The model under review builds one solid part; all positions refer to its coordinate system, in mm. Face numbers are marked on the shaded views. A direction names the side the tool comes from. Give positions to 0.01 mm unless a question says otherwise; leave off trailing zeros. Loops run counter-clockwise (first coordinate to the right, second up) from the corner with the lowest first, then second, coordinate; pieces in that order, holes last. Notation, with made-up numbers: M 20,-20 L 35,-20 A24 ccw 35,-7 Z; hole C 40.25,-23.5 d10. An arc over 180 degrees is marked long. One line per item, written item: value. Start each with the question number.
Q1. For the marked faces 1, 2 and 3, list the 3-axis set-ups (+Z, -Z, +X, -X, +Y, -Y) from which the entire face can be reached by the end or side of a thin tool; tool diameter is ignored.
Q2. We need section A-A on x = -83. Write out the cut boundary in (y, z).
Q3. We need section B-B on y = 8. Write out the cut boundary in (x, z).
Q4. Mouldability with a two-part tool opening along Y and no side actions: class the marked faces 4, 5 and 6 as released by +Y, released by -Y, zero draft, split by the parting line, or undercut.
Q5. For pin 1 (8 mm diameter, centred on x = -107, z = -29, fed in from +Y); pin 2 (15.5 mm diameter, centred on y = -14, z = 3.5, fed in from +X); pin 3 (5.5 mm diameter, centred on y = -68.5, z = 13.5, fed in from +X), all flat-tipped, find the tip position at first contact; note any pin that passes through.
Q6. We need section D-D on x = -66.5. Write out the cut boundary in (y, z), plus the area to 3 significant figures.
Q7. We need section C-C on z = -4. Write out the cut boundary in (x, y).
Q8. To check wall thickness, follow line 1 along Z through (x, y) = (-26.5, 23.5); line 2 along X through (y, z) = (1, 17); line 3 along X through (y, z) = (-15.5, 6). State the ranges of each line that lie inside material, in increasing order. Write a range as from..to.
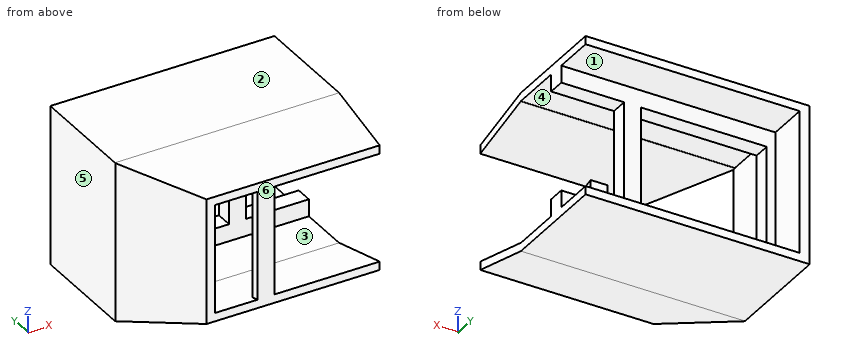
```python
from build123d import *

# Parameters (mm, degrees)
SKETCH1_W                = 74
SKETCH1_H                = 64
BOSS_EXTRUDE3_DEPTH      = 10
BOSS_EXTRUDE4_DEPTH      = 24
BOSS_EXTRUDE4_DEPTH_BACK = 80
SKETCH3_W                = 264
SKETCH3_H                = 94
SKETCH3_W_2              = 252.2
SKETCH3_H_2              = 84.2
SKETCH4_W                = 264
SKETCH4_H                = 94
SKETCH4_W_2              = 194
SKETCH4_H_2              = 64
BOSS_EXTRUDE5_DEPTH      = 40
CHAMFER4_SIZE            = 39.811344649
CHAMFER4_SIZE_2          = 30
CHAMFER7_SIZE            = 39.811344649
CHAMFER7_SIZE_2          = 30
CHAMFER8_SIZE            = 10
CHAMFER8_SIZE_2          = 40.107809335
CHAMFER9_SIZE            = 40.107809335
CHAMFER9_SIZE_2          = 10
SKETCH7_W                = 10
SKETCH7_H                = 74
BOSS_EXTRUDE6_DEPTH      = 5


with BuildPart() as part:
    # Sketch1 → Boss-Extrude3 (new body)
    with BuildSketch(Plane(origin=(0, 0, 0), x_dir=(1, 0, 0), z_dir=(0, 1, 0))):
        Polygon((-47, 42.1), (-126.1, 42.1), (-126.1, -42.1), (-47, -42.1), (-37, -42.1), (37, -42.1), (47, -42.1), (126.1, -42.1), (126.1, 42.1), (47, 42.1), (37, 42.1), (-37, 42.1), align=None)
        with Locations((-84, 0)):
            Rectangle(SKETCH1_W, SKETCH1_H, mode=Mode.SUBTRACT)
        Rectangle(SKETCH1_W, SKETCH1_H, mode=Mode.SUBTRACT)
        with Locations((84, 0)):
            Rectangle(SKETCH1_W, SKETCH1_H, mode=Mode.SUBTRACT)
    extrude(amount=BOSS_EXTRUDE3_DEPTH)

    # Sketch3 → Boss-Extrude4 (add, two sides: drawn at the far end of the back side and taken through both)
    with BuildSketch(Plane(origin=(0, 10, 0), x_dir=(1, 0, 0), z_dir=(0, 1, 0)).offset(-BOSS_EXTRUDE4_DEPTH_BACK)):
        Rectangle(SKETCH3_W, SKETCH3_H)
        Rectangle(SKETCH3_W_2, SKETCH3_H_2, mode=Mode.SUBTRACT)
    extrude(amount=BOSS_EXTRUDE4_DEPTH + BOSS_EXTRUDE4_DEPTH_BACK)

    # Sketch4 → Boss-Extrude5 (add)
    with BuildSketch(Plane(origin=(0, -70, 0), x_dir=(-1, 0, 0), z_dir=(0, -1, 0))):
        Rectangle(SKETCH4_W, SKETCH4_H)
        Rectangle(SKETCH4_W_2, SKETCH4_H_2, mode=Mode.SUBTRACT)
    extrude(amount=-BOSS_EXTRUDE5_DEPTH)

    # Chamfer4
    # the kernel refuses this chamfer: 39.811344649, 30 mm, written as the material it takes off along each edge
    with BuildSketch(Plane(origin=(-132, -70, 149.735778307), x_dir=(-0.023321052992758384, 0.9997280272590686, 0), z_dir=(0, 0, -1))) as chamfer4_piece_1:
        Polygon((CHAMFER4_SIZE * 0.999728027249, CHAMFER4_SIZE * 0.0233210529925), (-CHAMFER4_SIZE_2 * 0.0233210529928, CHAMFER4_SIZE_2 * 0.999728027259), (0, 0), align=None)
    extrude(amount=299.471556613, mode=Mode.SUBTRACT)
    with BuildSketch(Plane(origin=(-97, -30, 32), x_dir=(-0.9991572559820394, 0.04104604510109794, 0), z_dir=(0, 0, -1))) as chamfer4_piece_2_section:
        Polygon((CHAMFER4_SIZE_2 * 0.999157255982, -CHAMFER4_SIZE_2 * 0.0410460451011), (-CHAMFER4_SIZE * 0.0410460451007, -CHAMFER4_SIZE * 0.999157255972), (0, 0), align=None)
    chamfer4_piece_2 = extrude(amount=64, mode=Mode.PRIVATE)
    chamfer4_piece_2 = split(chamfer4_piece_2, bisect_by=Plane(origin=(-126.1, -43.282043753, 0), z_dir=(1, 0, 0)), keep=Keep.TOP, mode=Mode.PRIVATE)
    add(chamfer4_piece_2, mode=Mode.SUBTRACT)

    # Chamfer7
    # the kernel refuses this chamfer: 39.811344649, 30 mm, written as the material it takes off along each edge
    with BuildSketch(Plane(origin=(132, -70, -149.735778307), x_dir=(0.02332105299275837, 0.9997280272590686, 0), z_dir=(0, 0, 1))) as chamfer7_piece_1:
        Polygon((CHAMFER7_SIZE * 0.999728027249, CHAMFER7_SIZE * 0.0233210529925), (-CHAMFER7_SIZE_2 * 0.0233210529928, CHAMFER7_SIZE_2 * 0.999728027259), (0, 0), align=None)
    extrude(amount=299.471556613, mode=Mode.SUBTRACT)
    with BuildSketch(Plane(origin=(97, -30, -32), x_dir=(0.9991572559820394, 0.04104604510109794, 0), z_dir=(0, 0, 1))) as chamfer7_piece_2_section:
        Polygon((CHAMFER7_SIZE_2 * 0.999157255982, -CHAMFER7_SIZE_2 * 0.0410460451011), (-CHAMFER7_SIZE * 0.0410460451007, -CHAMFER7_SIZE * 0.999157255972), (0, 0), align=None)
    chamfer7_piece_2 = extrude(amount=64, mode=Mode.PRIVATE)
    chamfer7_piece_2 = split(chamfer7_piece_2, bisect_by=Plane(origin=(126.1, -43.282043753, 0), z_dir=(-1, 0, 0)), keep=Keep.TOP, mode=Mode.PRIVATE)
    add(chamfer7_piece_2, mode=Mode.SUBTRACT)

    # Chamfer8
    # the kernel refuses this chamfer: 40.107809335, 10 mm, written as the material it takes off along each edge
    with BuildSketch(Plane(origin=(230.265686152, -30, -32), x_dir=(0, 0.14819517765013807, -0.9889581332499592), z_dir=(-1, 0, 0))) as chamfer8_piece_1_section:
        Polygon((CHAMFER8_SIZE * 0.98895813325, CHAMFER8_SIZE * 0.14819517765), (-CHAMFER8_SIZE_2 * 0.148195177651, CHAMFER8_SIZE_2 * 0.988958133259), (0, 0), align=None)
    chamfer8_piece_1 = extrude(amount=460.531372304, mode=Mode.PRIVATE)
    chamfer8_piece_1 = split(chamfer8_piece_1, bisect_by=Plane(origin=(97, -69.925531208, -32.022723521), z_dir=(-1, 0, 0)), keep=Keep.TOP, mode=Mode.PRIVATE)
    chamfer8_piece_1 = split(chamfer8_piece_1, bisect_by=Plane(origin=(-97, -69.925531208, -32.022723521), z_dir=(1, 0, 0)), keep=Keep.TOP, mode=Mode.PRIVATE)
    add(chamfer8_piece_1, mode=Mode.SUBTRACT)
    with BuildSketch(Plane(origin=(126.1, -30, -32), x_dir=(0, 0.14819517765040952, -0.9889581332499185), z_dir=(-1, 0, 0))) as chamfer8_piece_2_section:
        Polygon((CHAMFER8_SIZE * 0.98895813325, CHAMFER8_SIZE * 0.14819517765), (-CHAMFER8_SIZE_2 * 0.148195177652, CHAMFER8_SIZE_2 * 0.988958133259), (0, 0), align=None)
    chamfer8_piece_2 = extrude(amount=252.2, mode=Mode.PRIVATE)
    chamfer8_piece_2 = split(chamfer8_piece_2, bisect_by=Plane(origin=(115.387923489, -45.409746002, -35.753076102), z_dir=(-0.7986355100471506, 0.6018150231522371, 0)), keep=Keep.TOP, mode=Mode.PRIVATE)
    chamfer8_piece_2 = split(chamfer8_piece_2, bisect_by=Plane(origin=(-37.003214765, -149.429767809, -35.753076102), z_dir=(0.7986355100471506, 0.6018150231522371, 0)), keep=Keep.TOP, mode=Mode.PRIVATE)
    add(chamfer8_piece_2, mode=Mode.SUBTRACT)
    with BuildSketch(Plane(origin=(-206.165686152, -70, -47), x_dir=(0, 0.9999566151296001, -0.009314926653100013), z_dir=(1, 0, 0))) as chamfer8_piece_3:
        Polygon((CHAMFER8_SIZE_2 * 0.999956615139, CHAMFER8_SIZE_2 * 0.00931492665318), (-CHAMFER8_SIZE * 0.0093149266531, CHAMFER8_SIZE * 0.99995661513), (0, 0), align=None)
    extrude(amount=412.331372304, mode=Mode.SUBTRACT)

    # Chamfer9
    # the kernel refuses this chamfer: 40.107809335, 10 mm, written as the material it takes off along each edge
    with BuildSketch(Plane(origin=(-126.1, -30, 32), x_dir=(0, -0.9999566151296001, -0.009314926653099073), z_dir=(1, 0, 0))) as chamfer9_piece_1_section:
        Polygon((CHAMFER9_SIZE * 0.999956615139, -CHAMFER9_SIZE * 0.00931492665318), (-CHAMFER9_SIZE_2 * 0.00931492665339, -CHAMFER9_SIZE_2 * 0.99995661513), (0, 0), align=None)
    chamfer9_piece_1 = extrude(amount=252.2, mode=Mode.PRIVATE)
    chamfer9_piece_1 = split(chamfer9_piece_1, bisect_by=Plane(origin=(37.003214765, -149.429767809, 35.753076102), z_dir=(-0.7986355100471506, 0.6018150231522371, 0)), keep=Keep.TOP, mode=Mode.PRIVATE)
    chamfer9_piece_1 = split(chamfer9_piece_1, bisect_by=Plane(origin=(-115.387923489, -45.409746002, 35.753076102), z_dir=(0.79863551004721, 0.6018150231521583, 0)), keep=Keep.TOP, mode=Mode.PRIVATE)
    add(chamfer9_piece_1, mode=Mode.SUBTRACT)
    with BuildSketch(Plane(origin=(-230.265686152, -30, 32), x_dir=(0, -0.9999566151296001, -0.00931492665310001), z_dir=(1, 0, 0))) as chamfer9_piece_2_section:
        Polygon((CHAMFER9_SIZE * 0.999956615139, -CHAMFER9_SIZE * 0.00931492665318), (-CHAMFER9_SIZE_2 * 0.0093149266531, -CHAMFER9_SIZE_2 * 0.99995661513), (0, 0), align=None)
    chamfer9_piece_2 = extrude(amount=460.531372304, mode=Mode.PRIVATE)
    chamfer9_piece_2 = split(chamfer9_piece_2, bisect_by=Plane(origin=(97, -69.925531208, 32.022723521), z_dir=(-1, 0, 0)), keep=Keep.TOP, mode=Mode.PRIVATE)
    chamfer9_piece_2 = split(chamfer9_piece_2, bisect_by=Plane(origin=(-97, -69.925531208, 32.022723521), z_dir=(1, 0, 0)), keep=Keep.TOP, mode=Mode.PRIVATE)
    add(chamfer9_piece_2, mode=Mode.SUBTRACT)
    with BuildSketch(Plane(origin=(206.165686152, -70, 47), x_dir=(0, -0.1481951776501387, -0.9889581332499591), z_dir=(-1, 0, 0))) as chamfer9_piece_3:
        Polygon((CHAMFER9_SIZE_2 * 0.98895813325, -CHAMFER9_SIZE_2 * 0.14819517765), (-CHAMFER9_SIZE * 0.148195177651, -CHAMFER9_SIZE * 0.988958133259), (0, 0), align=None)
    extrude(amount=412.331372304, mode=Mode.SUBTRACT)

    # Split1
    split(bisect_by=Plane(origin=(0, 0, 0), x_dir=(0, 0, 1), z_dir=(1, 0, 0)), keep=Keep.BOTTOM)

    # Sketch7 → Boss-Extrude6 (add)
    with BuildSketch(Plane(origin=(0, -65, 0), x_dir=(-1, 0, 0), z_dir=(0, -1, 0))):
        with Locations((67, 0)):
            Rectangle(SKETCH7_W, SKETCH7_H)
    extrude(amount=BOSS_EXTRUDE6_DEPTH)


solid = part.part
```
Solved:
1. face 1: +X, +Y
1. face 2: +Z, +X, -X, +Y, -Y
1. face 3: +X
2. outline: M -70,-37 L -29.89,-47 L 34,-47 L 34,-42.1 L 10,-42.1 L 10,-32 L 0,-32 L 0,-42.1 L -30,-42.1 L -30,-42 L -70,-32.03 Z; M -70,32.03 L -30,42 L -30,42.1 L 0,42.1 L 0,32 L 10,32 L 10,42.1 L 34,42.1 L 34,47 L -29.89,47 L -70,37 Z
3. outline: M -132,-47 L 0,-47 L 0,-32 L -37,-32 L -37,32 L 0,32 L 0,47 L -132,47 Z; hole M -121,-32 L -47,-32 L -47,32 L -121,32 Z
4. face 4: undercut
4. face 5: zero draft
4. face 6: released by -Y
5. pin 1: y = 10
5. pin 2: x = -126.1
5. pin 3: x = -62
6. outline: M -70,-37 L -29.89,-47 L 34,-47 L 34,-42.1 L 10,-42.1 L 10,-32 L 0,-32 L 0,-42.1 L -30,-42.1 L -30,-42 L -65,-33.27 L -65,33.27 L -30,42 L -30,42.1 L 0,42.1 L 0,32 L 10,32 L 10,42.1 L 34,42.1 L 34,47 L -29.89,47 L -70,37 Z
6. area: 1,550 mm2
7. outline: M -132,-30.19 L -102,-70 L -97,-70 L -97,-69.81 L -126.1,-31.19 L -126.1,0 L -121,0 L -121,10 L -126.1,10 L -126.1,34 L -132,34 Z; M -72,-70 L -62,-70 L -62,-65 L -72,-65 Z; M -47,0 L -37,0 L -37,10 L -47,10 Z
8. line 1: -47..-42.1, 42.1..47
8. line 2: -132..-121, -47..-37
8. line 3: -132..-126.1
